Here's how the part is built. I have some questions about the finished solid (model axes, mm). A direction names the side the tool comes from. Round coordinates to 2 decimals unless told otherwise and drop trailing zeros. Write each loop counter-clockwise with the first axis right and the second up, starting at its lowest first coordinate (ties: lowest second). Pieces come first, ordered by that corner, then holes. Notation, with made-up numbers: (62.25, 80.25) - (101.25, 80.25) arc R5 ccw to (101.25, 87.25) - close; hole circle Ø4 at (69, 30). An arc over 180 degrees is marked (long way). One line per item, written item: value. Start each with the question number.
Item 1: Imagine slicing it at B-B, the plane z = -30. Please give me the cut outline in (x, y).
Item 2: For faces 4 (the face through (0.67, 0.986, -38.383)), 5 (the face through (0, 2, 42)), which set-ups out of +Z, -Z, +X, -X, +Y, -Y let a thin tool reach every point of the face, with its end or its side?
Item 3: If I drill on line 1 (Z direction, x = -0.25, y = 1.2); line 2 (Z direction, x = 0, y = 2.8); line 3 (X direction, y = 1.2, z = 0), over which ranges is the centre line in solid material (lowest first)?
Item 4: For P1, Ø1.8, axis at x = -1, z = -39.5, coming from the +Y side; P2, Ø0.6, axis at y = 4, z = 2.5, coming from the +X side; P3, Ø4, axis at x = 0, z = -40, coming from the -Y side; P4, Ø0.8, axis at y = 4, z = 21, coming from the -X side, each with a flat end and sliding along its axis, tell me the tip position at first contact or that it passes through.
Item 5: Thinking about a two-plate mould opening in Z: for faces 1 (the face through (2, 0, -1)), 2 (the face through (0, 3, 47.5)), 3 (the face through (0, 2, -38)), which applies, released by +Z, released by -Z, zero draft, split by the parting line, or undercut?
Item 6: Imagine slicing it at C-C, the plane x = 0. Count the separate pieces of the cut face and the enclosed holes in it, then the cut area to 4 significant figures.
Autodesk Inventor part; units mm, degrees
ref_plane "to_block_XY" through (0, 5.5, 0) normal (0, 0, 1) x (1, 0, 0)
ref_plane "to_block_YZ" through (0, 5.5, 0) normal (1, 0, 0) x (0, 1, 0)
ref_plane "to_block_ZX" through (0, 5.5, 0) normal (0, 1, 0) x (0, 0, 1)
sketch "Sketch_12" plane through (0, 0, 0) normal (0, 0, 1) x (1, 0, 0)
  line L0 (-4.5, 5.3) -> (-4.5, 5.0434)
  line L1 (-4.5, 5.0434) -> (-4.2216, 4.8827)
  arc A0 (-3.7548, 4.35) -> (-4.2216, 4.8827) centre (-4.7715, 3.93) ccw
  line L2 (-3.7548, 4.35) -> (-3.1, 4.35)
  line L3 (-3.1, 4.35) -> (-3.1, 3.65)
  line L4 (-3.1, 3.65) -> (-3.7548, 3.65)
  arc A1 (-4.2216, 3.1173) -> (-3.7548, 3.65) centre (-4.7715, 4.07) ccw
  line L5 (-4.2216, 3.1173) -> (-4.5, 2.9566)
  line L6 (-4.5, 2.9566) -> (-4.5, 0.3)
  line L7 (-4.5, 0.3) -> (-4.2, 0)
  line L8 (-4.2, 0) -> (4.2, 0)
  line L9 (4.2, 0) -> (4.5, 0.3)
  line L10 (4.5, 0.3) -> (4.5, 2.9566)
  line L11 (4.5, 2.9566) -> (4.2216, 3.1173)
  arc A2 (3.7548, 3.65) -> (4.2216, 3.1173) centre (4.7715, 4.07) ccw
  line L12 (3.7548, 3.65) -> (3.1, 3.65)
  line L13 (3.1, 3.65) -> (3.1, 4.35)
  line L14 (3.1, 4.35) -> (3.7548, 4.35)
  arc A3 (4.2216, 4.8827) -> (3.7548, 4.35) centre (4.7715, 3.93) ccw
  line L15 (4.2216, 4.8827) -> (4.5, 5.0434)
  line L16 (4.5, 5.0434) -> (4.5, 5.3)
  line L17 (4.5, 5.3) -> (4.3, 5.5)
  line L18 (4.3, 5.5) -> (-4.3, 5.5)
  line L19 (-4.3, 5.5) -> (-4.5, 5.3)
extrude "Extrusion1" add sketch "Sketch_12" along normal mid plane 95
sketch "Sketch2" plane through (-4.3, 5.5, 47.5) normal (0, 1, 0) x (1, 0, 0)
  point P0 (4.3, 87.5)
hole "Hole1" at (0, 5.5, -40) direction (0, -1, 0) diameter 3.5 depth 5.5 counterbore diameter 6 counterbore depth 3.5
pattern_linear "Rectangular Pattern1" count 5 spacing 20 along (0, 0, 1) of "Hole1"
ref_plane "to_block_XY" through (0, 5.5, 0) normal (0, 0, 1) x (1, 0, 0)
ref_plane "to_block_YZ" through (0, 5.5, 0) normal (1, 0, 0) x (0, 1, 0)
ref_plane "to_block_ZX" through (0, 5.5, 0) normal (0, 1, 0) x (0, 0, 1)
properties part number "SSEBZ-MX10-95_r"
Values follow:
1. outline: (-4.5, 0.3) - (-4.2, 0) - (4.2, 0) - (4.5, 0.3) - (4.5, 2.96) - (4.22, 3.12) arc R1.1 cw to (3.75, 3.65) - (3.1, 3.65) - (3.1, 4.35) - (3.75, 4.35) arc R1.1 cw to (4.22, 4.88) - (4.5, 5.04) - (4.5, 5.3) - (4.3, 5.5) - (-4.3, 5.5) - (-4.5, 5.3) - (-4.5, 5.04) - (-4.22, 4.88) arc R1.1 cw to (-3.75, 4.35) - (-3.1, 4.35) - (-3.1, 3.65) - (-3.75, 3.65) arc R1.1 cw to (-4.22, 3.12) - (-4.5, 2.96) - close
2. face 4: +Y, -Y
2. face 5: +Y
3. line 1: z = -47.5 to -41.73, -38.27 to -21.73, -18.27 to -1.73, 1.73 to 18.27, 21.73 to 38.27, 41.73 to 47.5
3. line 2: z = -47.5 to -43, -37 to -23, -17 to -3, 3 to 17, 23 to 37, 43 to 47.5
3. line 3: x = -4.5 to -1.75, 1.75 to 4.5
4. P1: stops at y = 2
4. P2: stops at x = 3.1
4. P3: stops at y = 0
4. P4: stops at x = -3.78
5. face 1: zero draft
5. face 2: released by +Z
5. face 3: undercut
6. separate pieces: 6
6. enclosed holes: 0
6. area: 382.5 mm^2
